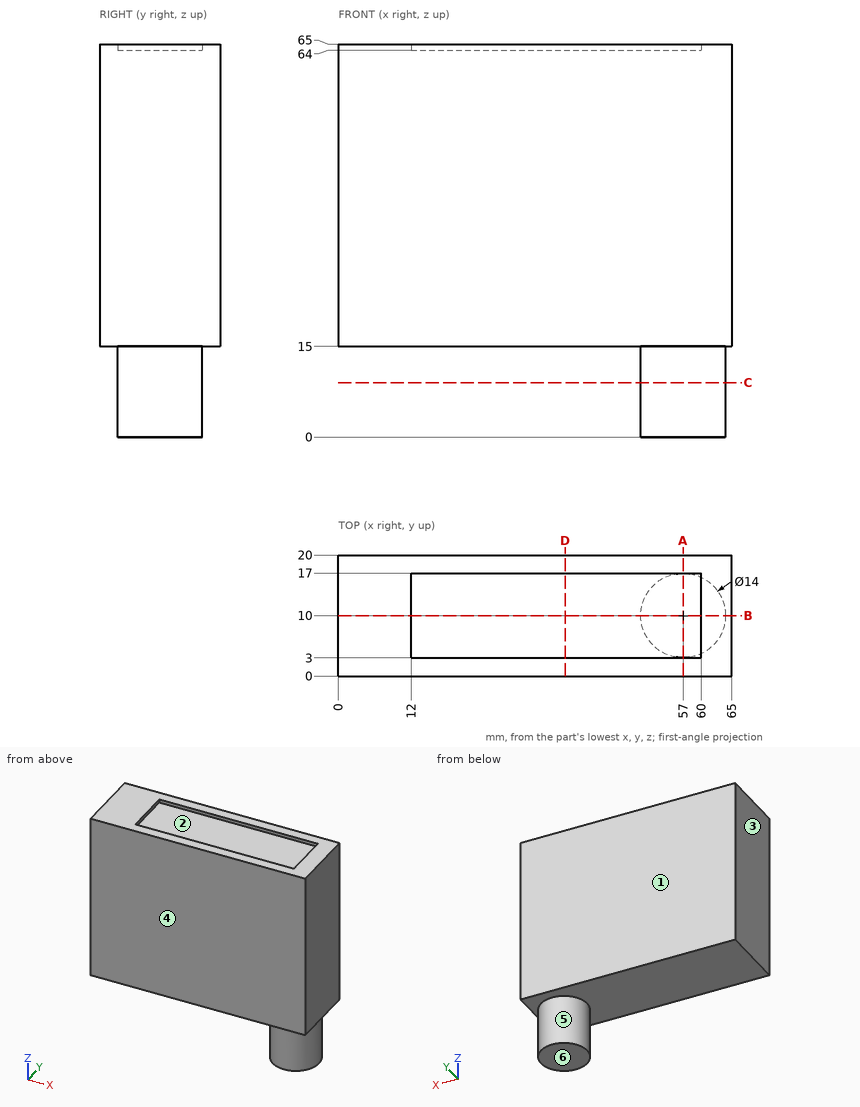
Design review of the part shown in the three views and the two pictorial views. Dimensions are in mm from the part's minimum x, y and z. A direction names the side the tool comes from. Give positions to 0.01 mm unless a question says otherwise; leave off trailing zeros. Write each loop counter-clockwise with the first axis right and the second up, starting at its lowest first coordinate (ties: lowest second). Pieces come first, ordered by that corner, then holes. Notation, with made-up numbers: (-39.5, 7) - (19.5, 7) arc R18 cw to (19.5, 18) - close; hole circle Ø1 at (-26.5, 67). An arc over 180 degrees is marked (long way). Return JSON: item names as keys, results as strings. Group by question number.
(1) Insertion check: pin 1 (12 mm diameter, centred on x = 11.5, y = 9, fed in from -Z); pin 2 (7 mm diameter, centred on x = 39, y = 10, fed in from +Z). Each pin has a flat end and moves straight along its axis. Give the tip position at first contact, or say it passes through.
(2) We need section D-D, the plane x = 37.5. Give the boundary of the cut face in (y, z).
(3) To check wall thickness, follow probe 1 along Z at (x, y) = (26, 10.5); probe 2 along Z at (x, y) = (51.5, 1.75); probe 3 along X at (y, z) = (7.25, 12). State the ranges of each line that lie inside material, in increasing order.
(4) We need section A-A, the plane x = 57. Give the boundary of the cut face in (y, z).
(5) We need section C-C, the plane z = 9. Give the boundary of the cut face in (x, y).
(6) We need section B-B, the plane y = 10. Give the boundary of the cut face in (x, z).
(7) Mouldability with a two-part tool opening along Y and no side actions: class the marked faces 1, 2, 3 and 4 as +Y half, -Y half, draft (parallel to the pull), parting line (faces both ways), or undercut.
(8) Machinability: for the marked faces 5 and 6, which of the approach directions +Z, -Z, +X, -X, +Y, -Y give a long, thin tool a straight path to every point of the face, cutting with its end or side? Answer none if there is none.
Reported:
{
 "1": {"pin 1": "stops at z = 15", "pin 2": "stops at z = 64"},
 "2": {"outline": "(0, 15) - (20, 15) - (20, 65) - (17, 65) - (17, 64) - (3, 64) - (3, 65) - (0, 65) - close"},
 "3": {"probe 1": "z = 15 to 64", "probe 2": "z = 15 to 65", "probe 3": "x = 50.56 to 63.44"},
 "4": {"outline": "(0, 15) - (3, 15) - (3, 0) - (17, 0) - (17, 15) - (20, 15) - (20, 65) - (17, 65) - (17, 64) - (3, 64) - (3, 65) - (0, 65) - close"},
 "5": {"outline": "circle Ø14 at (57, 10)"},
 "6": {"outline": "(0, 15) - (50, 15) - (50, 0) - (64, 0) - (64, 15) - (65, 15) - (65, 65) - (60, 65) - (60, 64) - (12, 64) - (12, 65) - (0, 65) - close"},
 "7": {"face 1": "+Y half", "face 2": "undercut", "face 3": "draft", "face 4": "-Y half"},
 "8": {"face 5": "-Z", "face 6": "-Z, +X, -X, +Y, -Y"}
}
